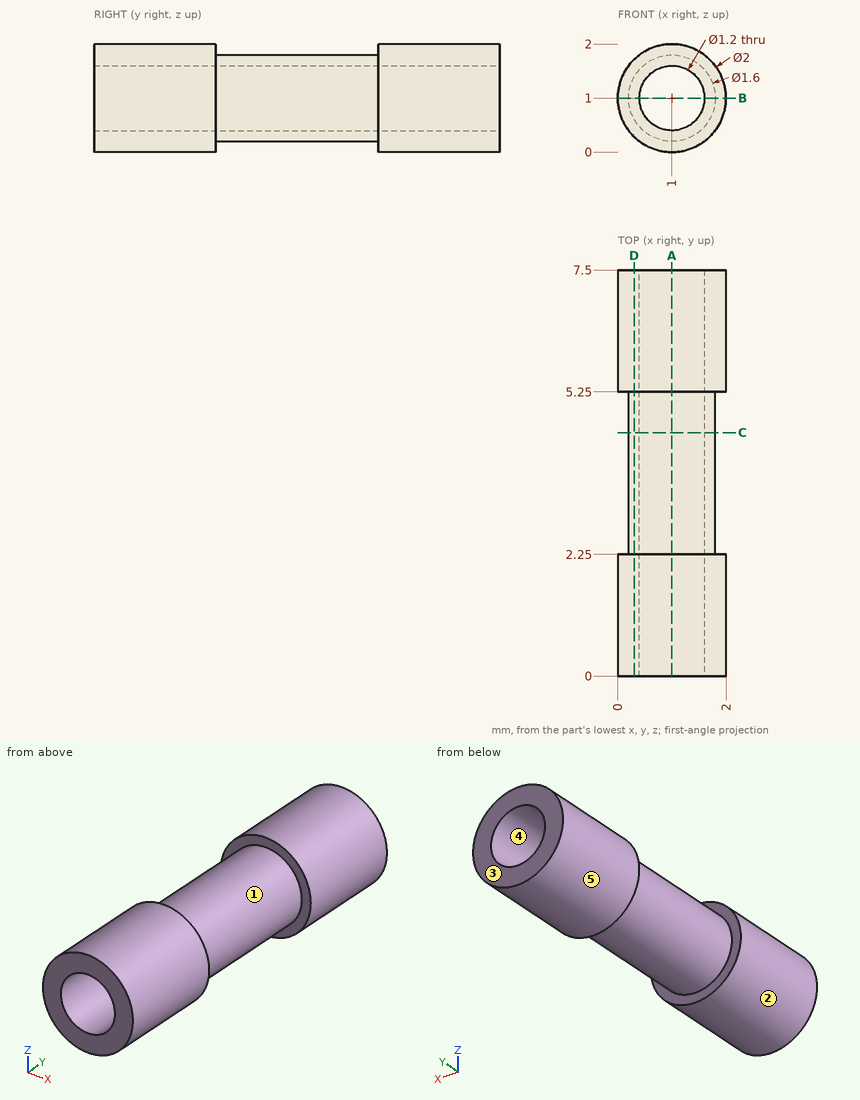
Input: dimensioned drawing with shaded views. Units: mm. Origin: part minimum x, y, z. A direction names the side the tool comes from. Give positions to 0.01 mm unless a question says otherwise; leave off trailing zeros. Write each loop counter-clockwise with the first axis right and the second up, starting at its lowest first coordinate (ties: lowest second). Pieces come first, ordered by that corner, then holes. Notation, with made-up numbers: (-8, 46) - (17, 46) arc R16 ccw to (17, 63) - close; hole circle Ø6 at (0, 10.25). An arc over 180 degrees is marked (long way). One line per item, written item: value. Start each with the question number.
Q1. Section query B-B, the plane z = 1. Return the cut outline in (x, y), then the cut area to 3 significant figures.
Q2. Material intervals for probe 1 along Z at (x, y) = (1, 5.5); probe 2 along X at (y, z) = (3, 1); probe 3 along Y at (x, z) = (0.3, 1.55), sorted ascending. Write a range as from..to.
Q3. Section query D-D, the plane x = 0.3. Return the cut outline in (y, z).
Q4. Section query C-C, the plane y = 4.5. Return the cut outline in (x, z).
Q5. First-contact query: pin 1 Ø1 at (y, z) = (3, 0.5) entering from -X. Flat tip, straight axial feed; report the tip coordinate or a pass-through.
Q6. Draft query along Z for the marked faces 3, 4 and 5. Return one class per face: +Z half, -Z half, draft (parallel to the pull), parting line (faces both ways), or undercut.
Q7. Set-up query: the marked faces 1 and 2. Return all of +Z, -Z, +X, -X, +Y, -Y with unobstructed straight access to the full face (end or side cutting, diameter ignored); none if empty.
Q8. Section query A-A, the plane x = 1. Return the cut outline in (y, z).
Answer:
1. outline: (0, 0) - (0.4, 0) - (0.4, 7.5) - (0, 7.5) - (0, 5.25) - (0.2, 5.25) - (0.2, 2.25) - (0, 2.25) - close; (1.6, 0) - (2, 0) - (2, 2.25) - (1.8, 2.25) - (1.8, 5.25) - (2, 5.25) - (2, 7.5) - (1.6, 7.5) - close
1. area: 4.80 mm2
2. probe 1: z = 0..0.4, 1.6..2
2. probe 2: x = 0.2..0.4, 1.6..1.8
2. probe 3: y = 0..2.25, 5.25..7.5
3. outline: (0, 0.29) - (2.25, 0.29) - (2.25, 0.61) - (5.25, 0.61) - (5.25, 0.29) - (7.5, 0.29) - (7.5, 1.71) - (5.25, 1.71) - (5.25, 1.39) - (2.25, 1.39) - (2.25, 1.71) - (0, 1.71) - close
4. outline: circle Ø1.6 at (1, 1); hole circle Ø1.2 at (1, 1)
5. pin 1: stops at x = 0.2
6. face 3: draft
6. face 4: undercut
6. face 5: parting line
7. face 1: none
7. face 2: +Y, -Y
8. outline: (0, 0) - (2.25, 0) - (2.25, 0.2) - (5.25, 0.2) - (5.25, 0) - (7.5, 0) - (7.5, 0.4) - (0, 0.4) - close; (0, 1.6) - (7.5, 1.6) - (7.5, 2) - (5.25, 2) - (5.25, 1.8) - (2.25, 1.8) - (2.25, 2) - (0, 2) - close
